Input: part model. Units: mm. Frame: model coordinates. Coordinates: 2 decimals unless noted, no trailing zeros. Order: outer loops, then holes, each group sorted by start corner. A loop starts at its lowest first (then second) coordinate and runs counter-clockwise, first axis right, second up. Notation, with made-up numbers: (-8.5, -7.5) -> (37.5, -7.5) arc R23 ccw to (37.5, 1.5) -> close; hole circle Ø7 at (-30, -14.75). An arc over 180 degrees is marked (long way). Answer as CSV lines item,"result".
Autodesk Inventor part; units mm, degrees
ref_plane "YZ Plane" through (0, 0, 0) normal (1, 0, 0) x (0, 1, 0)
ref_plane "XZ Plane" through (0, 0, 0) normal (0, 1, 0) x (-1, 0, 0)
ref_plane "XY Plane" through (0, 0, 0) normal (0, 0, 1) x (1, 0, 0)
sketch "Skizze1" plane through (0, 0, 0) normal (0, 1, 0) x (-1, 0, 0)
  line L0 (0, 0) -> (3.5, 0)
  line L1 (3.5, 0) -> (3.5, -0.75)
  line L2 (3.5, -0.75) -> (2.5, -0.75)
  line L3 (2.5, -0.75) -> (2.5, -4.25)
  line L4 (0, -6.75) -> (0, -6.75)
  line L5 (0, -6.75) -> (0, 0)
  arc A0 (0, -6.75) -> (2.5, -4.25) centre (0, -4.25) ccw
  point P0 (2.5, -6.75)
  dimension "d6" = 3.5
  dimension "d7" = 0.75
  dimension "d8" = 1
  dimension "d9" = 6
  dimension "d10" = 2.5
revolve "Umdrehung1" add sketch "Skizze1" angle 360 about axis through (0, 0, -6.75) along (0, 0, 1)
sketch "Skizze2" plane through (0, 0, 0) normal (0, 0, 1) x (1, 0, 0)
  circle A0 centre (0, 0) radius 3.5
  circle A1 centre (0, 0) radius 3.5
  circle A2 centre (-1.27, 0) radius 0.25
  circle A3 centre (1.27, 0) radius 0.25
  point P0 (0, 0)
  dimension "d11" = 0.5
  dimension "d12" = 0.5
  dimension "d13" = 1.27
  dimension "d14" = 1.27
extrude "Extrusion1" add sketch "Skizze2" along normal blind 10 contours A2 | A3
properties part number "licht_led_gruen"
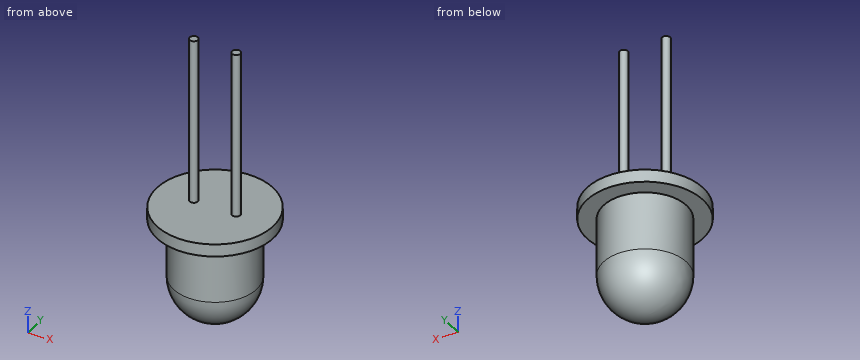
1. Ray query, line 1 along Z through (x, y) = (2.75, 0.25); line 2 along Z through (x, y) = (-0.25, 0.25); line 3 along X through (y, z) = (-1.75, -1). Return the intervals inside material, ascending.
Findings:
line 1,"z = -0.75 to 0"
line 2,"z = -6.72 to 0"
line 3,"x = -1.79 to 1.79"
2. Cut plane C-C (x = 0). Return the cut outline in (y, z), plus the area to 3 significant figures.
Findings:
outline,"(-3.5, -0.75) -> (-2.5, -0.75) -> (-2.5, -4.25) arc R2.5 ccw to (2.5, -4.25) -> (2.5, -0.75) -> (3.5, -0.75) -> (3.5, 0) -> (-3.5, 0) -> close"
area,"32.6 mm2"
3. Cut plane B-B (z = 4.5). Return the cut outline in (x, y), plus the area to 3 significant figures.
Findings:
outline,"circle Ø0.5 at (-1.27, 0); circle Ø0.5 at (1.27, 0)"
area,"0.393 mm2"
4. Cut plane A-A (y = 0). Return the cut outline in (x, z), plus the area to 3 significant figures.
Findings:
outline,"(-3.5, -0.75) -> (-2.5, -0.75) -> (-2.5, -4.25) arc R2.5 ccw to (2.5, -4.25) -> (2.5, -0.75) -> (3.5, -0.75) -> (3.5, 0) -> (1.52, 0) -> (1.52, 10) -> (1.02, 10) -> (1.02, 0) -> (-1.02, 0) -> (-1.02, 10) -> (-1.52, 10) -> (-1.52, 0) -> (-3.5, 0) -> close"
area,"42.6 mm2"
5. Contact query for flat-ended pins moving along their axis: pin 1 (3.5 mm diameter, centred on x = 1.5, y = -1.5, fed in from -Z); pin 2 (3 mm diameter, centred on y = 0, z = 2.5, fed in from -X); pin 3 (2 mm diameter, centred on x = -2, y = 0.5, fed in from -Z). Output: stop coordinate, or through.
Findings:
pin 1,"stops at z = -6.72"
pin 2,"stops at x = -1.52"
pin 3,"stops at z = -6.51"
6. Cut plane D-D (z = -1). Return the cut outline in (x, y).
Findings:
outline,"circle Ø5 at (0, 0)"
